Geometry: final body of the model. Coordinates: model frame, mm. Give positions to 0.01 mm unless a question says otherwise; leave off trailing zeros. Write each loop counter-clockwise with the first axis right and the second up, starting at its lowest first coordinate (ties: lowest second). Pieces come first, ordered by that corner, then holes. Notation, with made-up numbers: M 1.25,17 L 56.25,17 A20 cw 56.25,23 Z; hole C -17,-12.5 d1. An arc over 180 degrees is marked long. Use a Markdown table: item, result. Add a question column.
1) Section D-D on z = 61. Return the cut outline in (x, y).
2) Section C-C on z = 234. Return the cut outline in (x, y).
3) Pin query (flat end, axial travel): pin 1 (10 mm diameter, centred on x = 42.5, y = -12, fed in from +Z); pin 2 (1.5 mm diameter, centred on x = 29, y = 5, fed in from -Z); pin 3 (5 mm diameter, centred on y = 23.5, z = 133, fed in from -X). Return the tip coordinate at first contact, or that it passes through.
4) Section A-A on y = 0. Return the cut outline in (x, z).
5) Draft query along Y for faces 1 (the cylindrical face through (-58.454, -44.821, 164.389)), 2 (the flat face through (-39.9, 62.4, 254)), 3 (the conical face through (-4.95, -22.3, 22.84)). Return one class per face: +Y half, -Y half, draft (parallel to the pull), parting line (faces both ways), or undercut.
6) Line query: line 1 (Y direction, x = 0, z = 194); line 2 (X direction, y = -2, z = 53); line 3 (Y direction, x = 0, z = 15.25). Output: solid intervals per line, ascending.
```python
from build123d import *

# Parameters (mm, degrees)
F0_R     = 76.2
F1_DEPTH = 254
F2_SIZE  = 76.2
F4_T     = -2.54
F5_D     = 25.4


with BuildPart() as f1:
    # F0 (on Top) → F1 (new body)
    with BuildSketch(Plane.XY):
        Circle(F0_R)
    extrude(amount=F1_DEPTH)

    # F2
    f2_edges = [f1.edges().sort_by_distance(p)[0] for p in [
        (-76.2, 0, 0),
    ]]
    chamfer(f2_edges, length=F2_SIZE)

    # F4
    f4_openings = [f1.faces().sort_by_distance(p)[0] for p in [
        (0, 0, 254),
    ]]
    offset(amount=F4_T, openings=f4_openings)

    # F5 (through all)
    with Locations(Plane(origin=(0, 0, 0), x_dir=(1, 0, 0), z_dir=(0, 0, -1))):
        with Locations((0, 0)):
            Hole(F5_D / 2)


solid = f1.part
```
Found:
| question | item | result |
|---|---|---|
| 1 | outline | C 0,0 d122; hole C 0,0 d114.82 |
| 2 | outline | C 0,0 d152.4; hole C 0,0 d147.32 |
| 3 | pin 1 | z = 52.75 |
| 3 | pin 2 | z = 28.68 |
| 3 | pin 3 | x = -73.25 |
| 4 | outline | M -76.2,76.2 L -12.7,12.7 L -12.7,16.29 L -73.66,77.25 L -73.66,254 L -76.2,254 Z; M 12.7,12.7 L 76.2,76.2 L 76.2,254 L 73.66,254 L 73.66,77.25 L 12.7,16.29 Z |
| 5 | face 1 | undercut |
| 5 | face 2 | draft |
| 5 | face 3 | parting line |
| 6 | line 1 | -76.2 to -73.66, 73.66 to 76.2 |
| 6 | line 2 | -52.96 to -49.37, 49.37 to 52.96 |
| 6 | line 3 | -15.25 to -12.7, 12.7 to 15.25 |
